Could you check a few things on this model? Use its own coordinates, in mm. A direction names the side the tool comes from. Give positions to 0.01 mm unless a question says otherwise; leave off trailing zeros. Loops run counter-clockwise (first coordinate to the right, second up) from the corner with the lowest first, then second, coordinate; pieces in that order, holes last. Notation, with made-up numbers: (83, 88.5) -> (110, 88.5) arc R8 cw to (110, 102.5) -> close; hole circle Ø11 at (-2, 77). An arc over 180 degrees is marked (long way). Put each result on its own line as item: value.
```python
from build123d import *

# Parameters (mm, degrees)
FILLET1_R  = 25
FILLET11_R = 25


# Some blends are built 0.0001 mm under size
with BuildPart() as part:
    # Sketch1 → Revolve1 (revolve)
    with BuildSketch(Plane(origin=(0, 0, 0), x_dir=(0, 0, -1), z_dir=(1, 0, 0))):
        Polygon((0, 0), (5.540701052, 11.882071751), (5.540701052, 16.882071751), (25, 16.882071751), (25, 19.382071751), (5.540701052, 19.382071751), (5.540701052, 40), (0, 40), align=None)
    revolve(axis=Axis((0, 0, 0), (0, 1, 0)))

    # Fillet1
    # the kernel refuses this fillet: 25 mm, written as the material it adds along each edge
    with BuildSketch(Plane(origin=(0, 16.882071751, 0), x_dir=(0, 0, -1), z_dir=(1, 0, 0))) as fillet1_piece_1:
        with BuildLine():
            CenterArc((20.540701052, -25), FILLET1_R, 90, 36.869897646)
            Line((20.540701052, 0), (20.540701052, 0.5))
            Line((20.540701052, 0.5), (5.540701052, 0.5))
            Line((5.540701052, 0.5), (5.040701052, 0))
            ThreePointArc((5.040701052, 0), (5.040701052, -2.5), (5.240701052, -4.6))
            Line((5.240701052, -4.6), (5.540701052, -5))
        make_face()
    revolve(axis=Axis((0, 16.882071751, 0), (0, 1, 0)))

    # Fillet11
    fillet11_edges = [part.edges().sort_by_distance(p)[0] for p in [
        (0, 11.882071751, 5.540701052),
    ]]
    fillet(fillet11_edges, radius=FILLET11_R - 0.0001)  # a hair under: the kernel refuses the full size


solid = part.part
```
1. For faces 1 (the face through (-7.509, 18.15, -23.846)), 2 (the face through (-24, 16.882, 0)), 3 (the face through (-1.664, 29.835, -5.285)), which set-ups out of +Z, -Z, +X, -X, +Y, -Y let a thin tool reach every point of the face, with its end or its side?
Recorded:
face 1: +Y, -Y
face 2: -Y
face 3: +Y
2. I'm going to push flat-ended pins straight in: pin 1 (10 mm diameter, centred on x = -10.5, z = 3, fed in from +Y); pin 2 (10 mm diameter, centred on y = 18.5, z = -8.5, fed in from +X); pin 3 (1 mm diameter, centred on x = 5, y = 28, fed in from +Z); pin 4 (5 mm diameter, centred on y = 7, z = 10, fed in from -X). Where does each tip first touch, or does it pass through?
Recorded:
pin 1: stops at y = 19.38
pin 2: stops at x = 24.75
pin 3: stops at z = 3.23
pin 4: passes through
3. I need wall thicknesses on line 1 (X direction, y = 25.5, z = 0.5); line 2 (Z direction, x = -3.5, y = 11); line 3 (Y direction, x = -9, z = 0). Which ranges of each line are inside material? Lowest first, please.
Recorded:
line 1: x = -5.52 to 5.52
line 2: z = -6.85 to 6.85
line 3: y = 12.03 to 19.38
4. If we section it at A-A (y = 21): List the corners of the cut face in (x, z) for me, then the cut area to 3 significant figures.
Recorded:
outline: circle Ø11.08 at (0, 0)
area: 96.4 mm^2
